Part print with two shaded views. Sizes in mm from the minimum x, y, z corner. A direction names the side the tool comes from. Coordinates: 2 decimals unless noted, no trailing zeros. Write each loop counter-clockwise with the first axis right and the second up, starting at its lowest first coordinate (ties: lowest second). Pieces come first, ordered by that corner, then holes.
Q1. Pin check, flat tips, straight feed: P1, Ø3, axis at x = 43, z = 2, coming from the +Y side; P2, Ø2, axis at x = 40, z = 9.5, coming from the -Y side; P3, Ø4, axis at x = 17, y = 9.5, coming from the +Z side. Stop position of each tip, or through.
Q2. Which spindle directions (+Z, -Z, +X, -X, +Y, -Y) get a long thin tool onto all of the face, cutting with end or side? Do the marked faces 1 and 2. Say none if no direction does.
Q3. Drill centre lines: probe 1 along Y at (x, z) = (25.4, 7.75) (1 decimal); probe 2 along Y at (x, z) = (25.4, 5.25); probe 3 along Z at (x, y) = (8.5, 22). Where is each one in solid material? Low to high.
Q4. Band-saw the part on C-C, the plane y = 18. Write the cut outline in (x, z) (3 decimals).
Q5. Pull direction Y, two halves, no side cores. Call the marked faces 3, 4 and 5: released by +Y, released by -Y, zero draft, split by the parting line, or undercut.
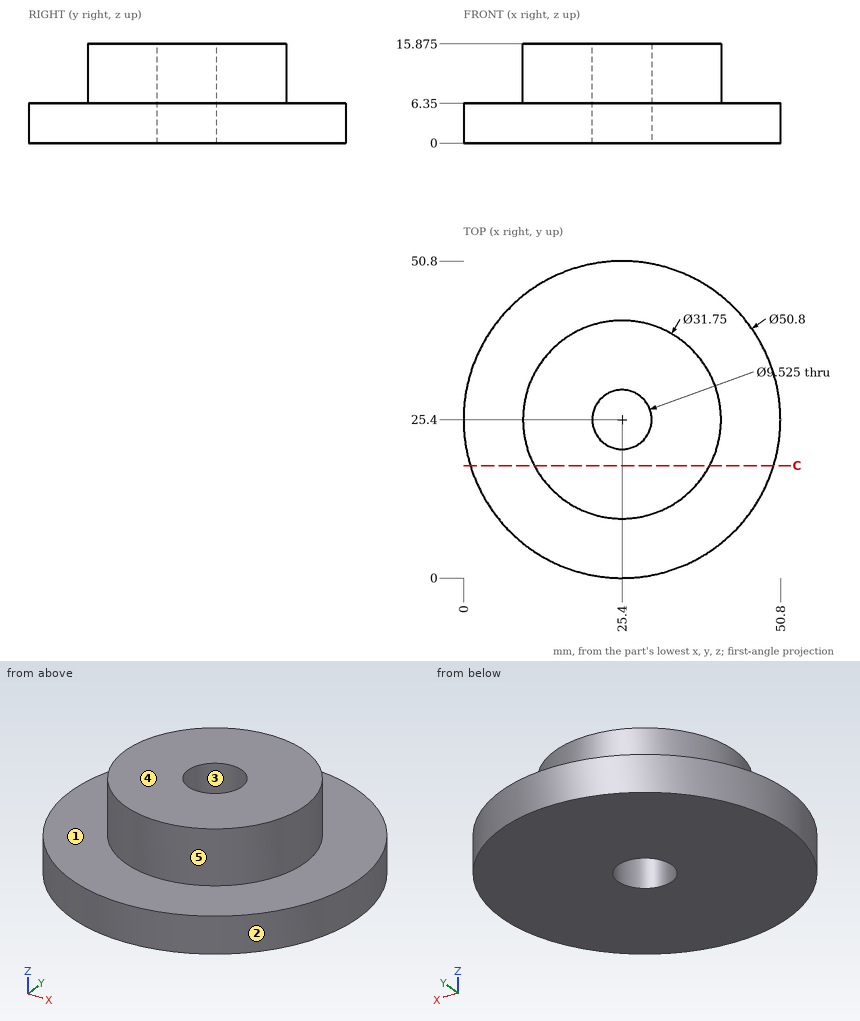
Answer sheet:
1. P1: stops at y = 45.05
1. P2: stops at y = 17.21
1. P3: stops at z = 6.35
2. face 1: +Z
2. face 2: +Z, -Z
3. probe 1: y = 9.5 to 20.6, 30.2 to 41.3
3. probe 2: y = 0 to 20.64, 30.16 to 50.8
3. probe 3: z = 0 to 6.35
4. outline: (1.102, 0) - (49.698, 0) - (49.698, 6.35) - (39.445, 6.35) - (39.445, 15.875) - (11.355, 15.875) - (11.355, 6.35) - (1.102, 6.35) - close
5. face 3: undercut
5. face 4: zero draft
5. face 5: split by the parting line
